Source: three-view drawing plus pictorial views. Frame: mm from the lowest corner of the part. Give positions to 0.01 mm unless a question says otherwise; leave off trailing zeros. Order: outer loops, then holes, each group sorted by start corner. A loop starts at its lowest first (then second) coordinate and runs counter-clockwise, first axis right, second up.
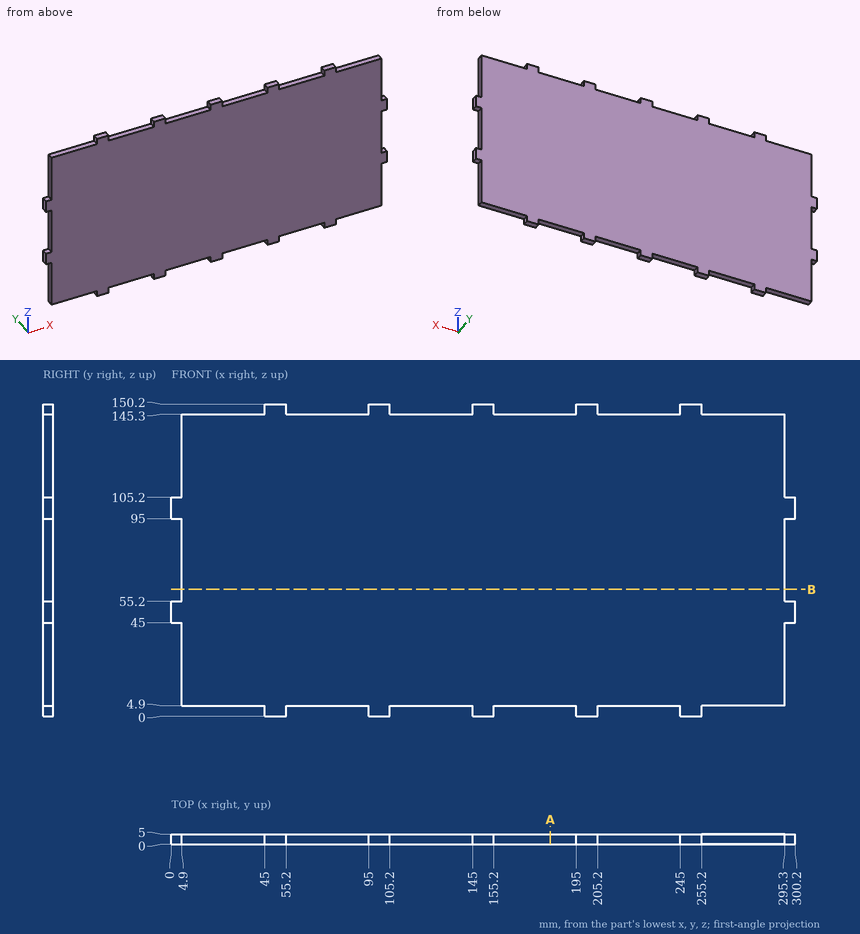
1) First-contact query: pin 1 Ø2.5 at (y, z) = (2.5, 147) entering from +X; pin 2 Ø1.5 at (x, y) = (116.5, 3.5) entering from +Z; pin 3 Ø3 at (x, y) = (158.5, 2.5) entering from -Z. Flat tips, straight axial feed; report the tip coordinate or a pass-through.
Checks:
pin 1: stops at x = 255.2
pin 2: stops at z = 145.3
pin 3: stops at z = 4.9
2) Ray query, L1, parallel to Z at x = 213, y = 1.8; L2, parallel to X at y = 2.9, z = 8. Return the intervals inside material, ascending.
Checks:
L1: z = 4.9 to 145.3
L2: x = 4.9 to 295.3
3) Section query B-B on z = 61. Output: boundary loops of the cut face in (x, y), and give its area (3 significant figures).
Checks:
outline: (4.9, 0) - (295.3, 0) - (295.3, 5) - (4.9, 5) - close
area: 1,450 mm2
4) Section query A-A on x = 182.5. Output: boundary loops of the cut face in (y, z), and give its area (3 significant figures).
Checks:
outline: (0, 4.9) - (5, 4.9) - (5, 145.3) - (0, 145.3) - close
area: 702 mm2
